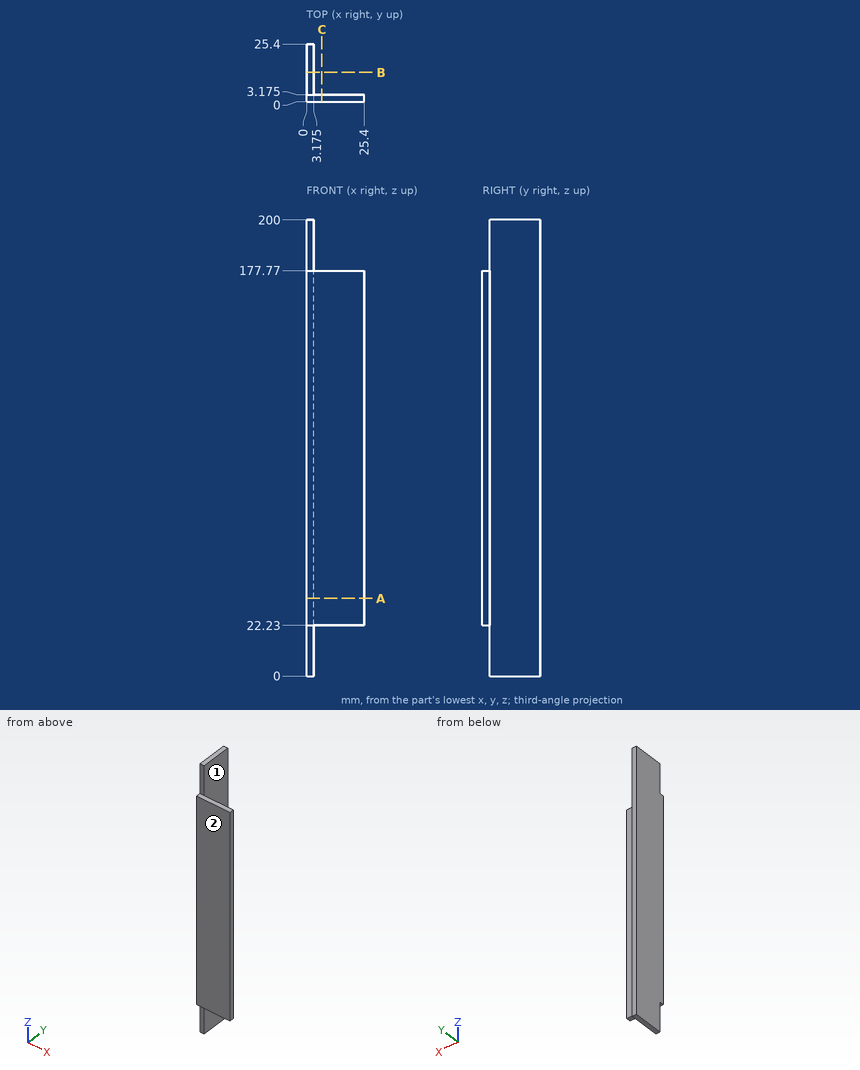
The figure shows three views and two pictorial views of one solid part (mm, origin at its lowest corner). Answer the questions. A direction names the side the tool comes from. Give positions to 0.01 mm unless a question says otherwise; leave off trailing zeros. Write each loop counter-clockwise with the first axis right and the second up, starting at its lowest first coordinate (ties: lowest second). Pieces come first, ordered by that corner, then holes. Notation, with made-up numbers: (66, 66) - (86, 66) arc R26 ccw to (86, 95) - close; hole circle Ø2 at (84.25, 20). An arc over 180 degrees is marked (long way). Use one line per item in the form item = value.
1. A cutting plane is placed at C-C (x = 6.75). Write down the section's boundary in (y, z) (3 decimals), and give its area (3 significant figures).
Filled in:
outline = (0, 22.23) - (3.175, 22.23) - (3.175, 177.77) - (0, 177.77) - close
area = 494 mm^2
2. Each of these flat-tipped pins is pushed along its axis until it touches: pin 1 Ø2.5 at (x, z) = (1.5, 12.5) entering from -Y (3 decimals); pin 2 Ø8 at (x, y) = (20, 6.5) entering from -Z; pin 3 Ø3.5 at (x, y) = (7.5, 1.5) entering from +Z. Where does it stop, or does it pass through?
Filled in:
pin_1 = 3.175
pin_2 = 22.23
pin_3 = 177.77
3. A cutting plane is placed at B-B (y = 13). Write down the section's boundary in (x, z) (3 decimals).
Filled in:
outline = (0, 0) - (3.175, 0) - (3.175, 200) - (0, 200) - close
4. Consider L1, parallel to Y at x = 16, z = 148 (3 decimals). Determine where the line is inside the solid, lowest interval first.
Filled in:
L1 = 0 to 3.175
5. A cutting plane is placed at A-A (z = 34). Write down the section's boundary in (x, y) (3 decimals).
Filled in:
outline = (0, 0) - (25.4, 0) - (25.4, 3.175) - (3.175, 3.175) - (3.175, 25.4) - (0, 25.4) - close
6. For the marked faces 1 and 2, determine the directions among +Z, -Z, +X, -X, +Y, -Y from which every point of the face is accessible in a straight line to the end or side of a thin tool.
Filled in:
face_1 = +Z, -Z, +X, +Y
face_2 = +Z, -Z, +X, -X, -Y
